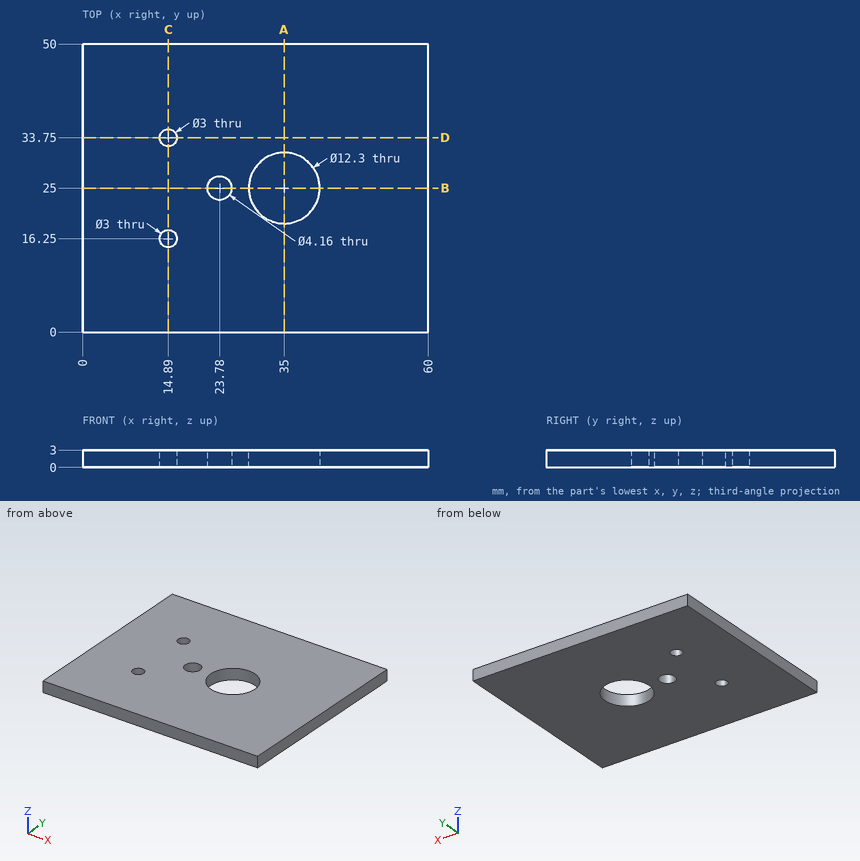
Check sheet for the drawn part. Datum: minimum x, y, z corner. Units: mm. Round coordinates to 2 decimals unless told otherwise and drop trailing zeros. Loops run counter-clockwise (first coordinate to the right, second up) from the corner with the lowest first, then second, coordinate; pieces in that order, holes last.
Item 1: Cross-section at B-B on y = 25. Record the boundary of the cut face in (x, z), then the cut area to 3 significant figures.
Item 2: Gauge pin test, flat ends, axial feed: pin 1 (2.5 mm diameter, centred on x = 14.89, y = 16.25, fed in from -Z); pin 2 (5 mm diameter, centred on x = 39, y = 26.5, fed in from +Z). Record the tip position at first contact, or that the pin passes through.
Item 3: Cross-section at A-A on x = 35. Record the boundary of the cut face in (y, z).
Item 4: Cross-section at D-D on y = 33.75. Record the boundary of the cut face in (x, z).
Item 5: Cross-section at C-C on x = 14.89. Record the boundary of the cut face in (y, z), then the cut area to 3 significant figures.
Item 6: Thickness scan on line 1 (Y direction, x = 14.89, z = 1); line 2 (Y direction, x = 23.78, z = 2.25); line 3 (Y direction, x = 35, z = 1.4). Record the ranges inside material, lowest first.
Answer sheet:
1. outline: (0, 0) - (21.7, 0) - (21.7, 3) - (0, 3) - close; (25.86, 0) - (28.85, 0) - (28.85, 3) - (25.86, 3) - close; (41.15, 0) - (60, 0) - (60, 3) - (41.15, 3) - close
1. area: 131 mm2
2. pin 1: passes through
2. pin 2: stops at z = 3
3. outline: (0, 0) - (18.85, 0) - (18.85, 3) - (0, 3) - close; (31.15, 0) - (50, 0) - (50, 3) - (31.15, 3) - close
4. outline: (0, 0) - (13.39, 0) - (13.39, 3) - (0, 3) - close; (16.39, 0) - (60, 0) - (60, 3) - (16.39, 3) - close
5. outline: (0, 0) - (14.75, 0) - (14.75, 3) - (0, 3) - close; (17.75, 0) - (32.25, 0) - (32.25, 3) - (17.75, 3) - close; (35.25, 0) - (50, 0) - (50, 3) - (35.25, 3) - close
5. area: 132 mm2
6. line 1: y = 0 to 14.75, 17.75 to 32.25, 35.25 to 50
6. line 2: y = 0 to 22.92, 27.08 to 50
6. line 3: y = 0 to 18.85, 31.15 to 50
